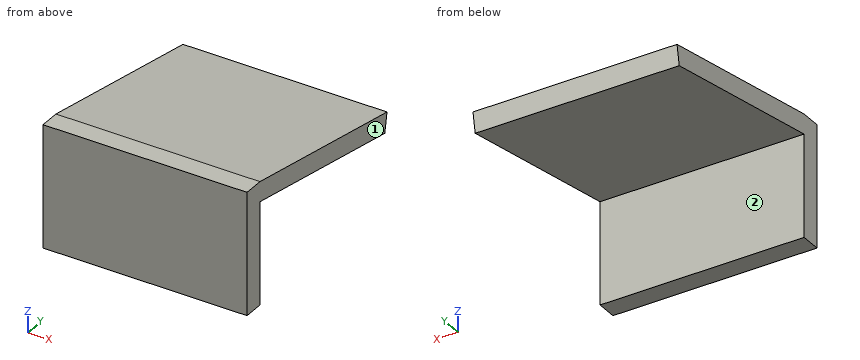
from build123d import *

# Parameters (mm, degrees)
SKETCH1_W           = 25
SKETCH1_H           = 15
BOSS_EXTRUDE1_DEPTH = 2.5
BOSS_EXTRUDE2_DEPTH = 25


with BuildPart() as part:
    # Sketch1 → Boss-Extrude1 (new body)
    with BuildSketch(Plane(origin=(0, 0, 0), x_dir=(1, 0, 0), z_dir=(0, 1, 0))):
        Rectangle(SKETCH1_W, SKETCH1_H)
    extrude(amount=BOSS_EXTRUDE1_DEPTH)

    # Sketch2 → Boss-Extrude2 (add, through all)
    with BuildSketch(Plane.ZY.offset(12.5)):
        Polygon((0.785626796, 26.701740143), (3.158795558, 27.120193825), (7.5, 2.5), (5.126831238, 2.081546317), align=None)
    extrude(amount=-BOSS_EXTRUDE2_DEPTH)


solid = part.part
The listing builds one solid part. Answer for the finished solid, in the listing's coordinates (mm). Face numbers are marked on the shaded views. A direction names the side the tool comes from. Round coordinates to 2 decimals unless told otherwise and drop trailing zeros. Write each loop counter-clockwise with the first axis right and the second up, starting at its lowest first coordinate (ties: lowest second). Pieces come first, ordered by that corner, then holes. Notation, with made-up numbers: M 18.5,7 L 49.5,7 A27 ccw 49.5,44 Z; hole C 22.5,27 d8. An arc over 180 degrees is marked long. Write each question's results on one line, items separated by ' | '. Start each with the question number.
Item 1: Find section B-B on z = 4.25. Write down the section's boundary in (x, y), and give its area (3 significant figures).
Item 2: Which of the six approach directions +Z, -Z, +X, -X, +Y, -Y give full straight-line access (tool end or side, diameter ignored) to the marked faces 1 and 2?
Item 3: Given pin 1 Ø3 at (x, y) = (-3.5, 5) entering from -Z; pin 2 Ø12 at (x, y) = (-1, 10) entering from +Z; pin 3 Ø4 at (x, z) = (-6, -2) entering from +Y, each flat-ended and moving along its own axis, determine where each tip first touches the part or whether it passes through.
Item 4: Find section D-D on z = -3.5. Write down the section's boundary in (x, y), and give its area (3 significant figures).
Item 5: Straight lines are drawn through the part: probe 1 along Y at (x, z) = (11, -2.25); probe 2 along Z at (x, y) = (10.5, 7); probe 3 along Z at (x, y) = (-1.5, 5.5). For each, find the intervals that lie inside material, in ascending order.
Item 6: Find section A-A on x = -8.25. Write down the section's boundary in (y, z), and give its area (3 significant figures).
Item 7: Find section C-C on z = 2.5. Write down the section's boundary in (x, y), and give its area (3 significant figures).
Answer block:
1) outline: M -12.5,0 L 12.5,0 L 12.5,2.5 L -12.5,2.5 Z; M -12.5,7.05 L 12.5,7.05 L 12.5,20.93 L -12.5,20.93 Z | area: 409 mm²
2) face 1: +Z, -Z, +X, +Y, -Y | face 2: -Z, +X, -X
3) pin 1: stops at z = 4.35 | pin 2: stops at z = 7.24 | pin 3: stops at y = 2.5
4) outline: M -12.5,0 L 12.5,0 L 12.5,2.5 L -12.5,2.5 Z | area: 62.5 mm²
5) probe 1: y = 0 to 2.5 | probe 2: z = 4.26 to 6.71 | probe 3: z = 4.52 to 6.97
6) outline: M 0,-7.5 L 2.5,-7.5 L 2.5,5.05 L 26.7,0.79 L 27.12,3.16 L 2.5,7.5 L 0,7.5 Z | area: 97.2 mm²
7) outline: M -12.5,0 L 12.5,0 L 12.5,2.5 L -12.5,2.5 Z; M -12.5,16.98 L 12.5,16.98 L 12.5,27 L -12.5,27 Z | area: 313 mm²
